The listing builds one solid part. Answer for the finished solid, in the listing's coordinates (mm). Face numbers are marked on the shaded views. A direction names the side the tool comes from. Round coordinates to 2 decimals unless told otherwise and drop trailing zeros. Order: outer loops, then holes, each group sorted by start corner. A loop starts at its lowest first (then second) coordinate and runs counter-clockwise, first axis right, second up. Notation, with made-up numbers: M 4.5,-40 L 17.5,-40 A25 cw 17.5,-28 Z; hole C 22.25,18 d10. An arc over 180 degrees is marked long. Write item = value, one per line. Start each with the question number.
(1) A cutting plane is placed at A-A, the plane z = 20. Determine the outline of the cut face in (x, y).
(2) Which of the six approach directions +Z, -Z, +X, -X, +Y, -Y give full straight-line access (tool end or side, diameter ignored) to the marked faces 4 and 5?
(3) A cutting plane is placed at C-C, the plane z = 8.5. Determine the outline of the cut face in (x, y).
(4) Straight lines are drawn through the part: probe 1 along Y at (x, z) = (63.1, 20); probe 2 along X at (y, z) = (0.5, 11.25); probe 3 along Y at (x, z) = (0, 1.55). For each, find the intervals that lie inside material, in ascending order. Write a range as from..to.
(5) For a pull along X with two mould halves and no side action, classify the marked faces 1, 2 and 3 as released by +X, released by -X, zero draft, split by the parting line, or undercut.
(6) A cutting plane is placed at D-D, the plane y = -13. Determine the outline of the cut face in (x, z).
(7) Each of these flat-tipped pins is pushed along its axis until it touches: pin 1 (2 mm diameter, centred on x = 26, z = 5.5, fed in from -Y); pin 2 (21 mm diameter, centred on x = 29.5, y = 8.5, fed in from +Z); pin 3 (5.5 mm diameter, centred on x = 6, z = 3, fed in from +Y); pin 4 (3.5 mm diameter, centred on y = -25, z = 20, fed in from +X). Where does it stop, or does it pass through?
(8) A cutting plane is placed at B-B, the plane y = 25. Determine the outline of the cut face in (x, z), and give its area (3 significant figures).
from build123d import *

# Parameters (mm, degrees)
BOSS_EXTRUDE1_DEPTH = 35
SKETCH2_W           = 100
SKETCH2_H           = 15
CUT_EXTRUDE1_DEPTH  = 5
SKETCH3_R           = 3
CUT_EXTRUDE2_DEPTH  = 138.931142241
SKETCH4_R           = 8
CUT_EXTRUDE3_DEPTH  = 3


with BuildPart() as part:
    # Sketch1 → Boss-Extrude1 (new, symmetric)
    with BuildSketch(Plane(origin=(0, 0, 0), x_dir=(1, 0, 0), z_dir=(0, 1, 0))):
        Polygon((0, 0), (65, 0), (65, -30), (60, -30), (60, -5), (0, -5), (-60, -5), (-60, -30), (-65, -30), (-65, 0), align=None)
    extrude(amount=BOSS_EXTRUDE1_DEPTH, both=True)

    # Sketch2 → Cut-Extrude1 (cut)
    with BuildSketch(Plane(origin=(0, 0, 0), x_dir=(-1, 0, 0), z_dir=(0, 0, -1))):
        with Locations((0, -27.5)):
            Rectangle(SKETCH2_W, SKETCH2_H)
        with Locations((0, 27.5)):
            Rectangle(SKETCH2_W, SKETCH2_H)
    extrude(amount=-CUT_EXTRUDE1_DEPTH, mode=Mode.SUBTRACT)

    # Sketch3 → Cut-Extrude2 (cut, through all)
    with BuildSketch(Plane.ZY.offset(65)):
        with Locations((20, 25)):
            Circle(SKETCH3_R)
        with Locations(Location((20, -25, 0), (0, 0, 180))):
            Circle(SKETCH3_R)
    extrude(amount=-CUT_EXTRUDE2_DEPTH, mode=Mode.SUBTRACT)

    # Sketch4 → Cut-Extrude3 (cut)
    with BuildSketch(Plane(origin=(0, 0, 0), x_dir=(-1, 0, 0), z_dir=(0, 0, -1))):
        Circle(SKETCH4_R)
    extrude(amount=-CUT_EXTRUDE3_DEPTH, mode=Mode.SUBTRACT)


solid = part.part
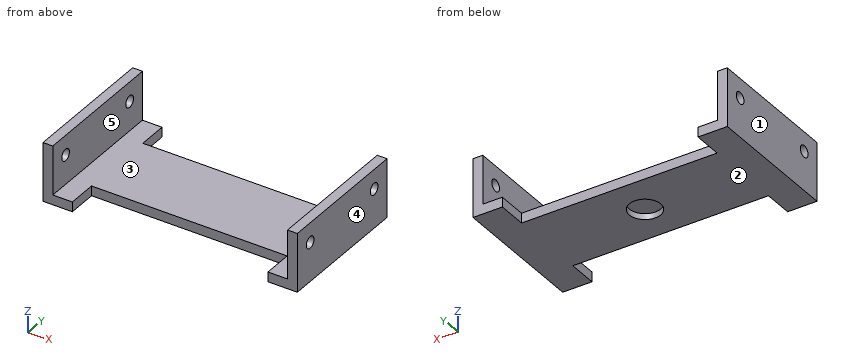
Reported:
q1.outline = M -65,-35 L -60,-35 L -60,-28 L -65,-28 Z; M -65,-22 L -60,-22 L -60,22 L -65,22 Z; M -65,28 L -60,28 L -60,35 L -65,35 Z; M 60,-35 L 65,-35 L 65,-28 L 60,-28 Z; M 60,-22 L 65,-22 L 65,22 L 60,22 Z; M 60,28 L 65,28 L 65,35 L 60,35 Z
q2.face_4 = +Z, -Z, +X, +Y, -Y
q2.face_5 = +Z, +Y, -Y
q3.outline = M -65,-35 L -60,-35 L -60,35 L -65,35 Z; M 60,-35 L 65,-35 L 65,35 L 60,35 Z
q4.probe_1 = -35..-28, -22..22, 28..35
q4.probe_2 = -65..-60, 60..65
q4.probe_3 = -20..-8, 8..20
q5.face_1 = released by -X
q5.face_2 = zero draft
q5.face_3 = undercut
q6.outline = M -65,0 L 65,0 L 65,30 L 60,30 L 60,5 L -60,5 L -60,30 L -65,30 Z
q7.pin_1 = -20
q7.pin_2 = 5
q7.pin_3 = 20
q7.pin_4 = through
q8.outline = M -65,0 L -50,0 L -50,5 L -60,5 L -60,17 L -65,17 Z; M -65,23 L -60,23 L -60,30 L -65,30 Z; M 50,0 L 65,0 L 65,17 L 60,17 L 60,5 L 50,5 Z; M 60,23 L 65,23 L 65,30 L 60,30 Z
q8.area = 340 mm²
